```python
from build123d import *

# Parameters (mm, degrees)
SKETCH2_R           = 6.35
BOSS_EXTRUDE1_DEPTH = 19.05
SKETCH3_R           = 3.175
CUT_EXTRUDE1_DEPTH  = 20.05
SKETCH4_W           = 3.175
SKETCH4_H           = 0.79375
CHAMFER1_SIZE       = 0.396875
SKETCH5_W           = 3.020451336
SKETCH5_H           = 1.5875


with BuildPart() as part:
    # Sketch2 → Boss-Extrude1 (new body)
    with BuildSketch(Plane.XY):
        Circle(SKETCH2_R)
    extrude(amount=BOSS_EXTRUDE1_DEPTH)

    # Sketch3 → Cut-Extrude1 (cut, through all)
    with BuildSketch(Plane.XY.offset(19.05)):
        Circle(SKETCH3_R)
    extrude(amount=-CUT_EXTRUDE1_DEPTH, mode=Mode.SUBTRACT)

    # Sketch4 → Cut-Revolve1 (revolve, cut)
    with BuildSketch(Plane(origin=(0, 0, 0), x_dir=(1, 0, 0), z_dir=(0, 1, 0))):
        with Locations((6.329219641, -15.719425)):
            Rectangle(SKETCH4_W, SKETCH4_H)
        with Locations((6.329219641, -3.330575)):
            Rectangle(SKETCH4_W, SKETCH4_H)
    revolve(axis=Axis((0, 0, 19.05), (0, 0, -1)), mode=Mode.SUBTRACT)

    # Chamfer1
    chamfer1_edges = [part.edges().sort_by_distance(p)[0] for p in [
        (-6.35, 0, 0),
        (-6.35, 0, 19.05),
    ]]
    chamfer(chamfer1_edges, length=CHAMFER1_SIZE)

    # Sketch5 → Cut-Revolve2 (revolve, cut)
    with BuildSketch(Plane(origin=(0, 0, 0), x_dir=(1, 0, 0), z_dir=(0, 1, 0))):
        with Locations((6.35, -11.90625)):
            Rectangle(SKETCH5_W, SKETCH5_H)
        with Locations((6.35, -7.14375)):
            Rectangle(SKETCH5_W, SKETCH5_H)
    revolve(axis=Axis((0, 0, 19.05), (0, 0, -1)), mode=Mode.SUBTRACT)


solid = part.part
```
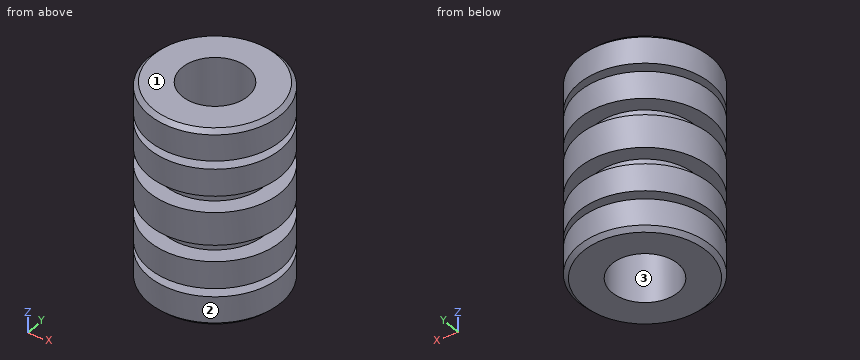
For this review, take the finished solid that the model builds, in its own axes (mm). Face numbers are marked on the shaded views. Round coordinates to 2 decimals unless told otherwise and drop trailing zeros. Write each loop counter-clockwise with the first axis right and the second up, starting at its lowest first coordinate (ties: lowest second). Pieces come first, ordered by that corner, then holes. Notation, with made-up numbers: (-15, 25.5) - (8, 25.5) arc R15 ccw to (8, 51.5) - close; hole circle Ø7 at (20, 41.5). An arc over 180 degrees is marked (long way). Answer as CSV lines item,"result". Start each with the question number.
(1) For pin 1 (3 mm diameter, centred on y = 2.5, z = 14, fed in from -X); pin 2 (1.5 mm diameter, centred on y = 4, z = 2.5, fed in from +X); pin 3 (1 mm diameter, centred on x = 5, z = 8.5, fed in from +Y), all flat-tipped, find the tip position at first contact; note any pin that passes through.
(2) Add section A-A, the plane z = 17.75. State the section outline as (x, y) points (3 decimals), plus the area to 3 significant figures.
(3) For line 1 (Z direction, x = 5.75, y = 1.5); line 2 (Y direction, x = 0, z = 15.25) (3 decimals); line 3 (Y direction, x = 0, z = 11.5) (3 decimals), list the stretches that pass through material, from the lowest coordinate up.
(4) Mouldability with a two-part tool opening along X and no side actions: class the marked faces 1, 2 and 3 as +X half, -X half, draft (parallel to the pull), parting line (faces both ways), or undercut.
(5) Add section B-B, the plane y = 5.25. State how many separate pieces and enclosed holes the cut face has, plus the area to 3 significant figures.
From the geometry:
1,pin 1,"stops at x = -6.27"
1,pin 2,"stops at x = 5.46"
1,pin 3,"stops at y = 4.48"
2,outline,"circle Ø12.7 at (0, 0); hole circle Ø6.35 at (0, 0)"
2,area,"95.0 mm²"
3,line 1,"z = 0 to 2.93, 3.73 to 6.35, 7.94 to 11.11, 12.7 to 15.32, 16.12 to 19.05"
3,line 2,"y = -6.35 to -3.175, 3.175 to 6.35"
3,line 3,"y = -4.84 to -3.175, 3.175 to 4.84"
4,face 1,"draft"
4,face 2,"parting line"
4,face 3,"undercut"
5,separate pieces,"5"
5,enclosed holes,"0"
5,area,"101 mm²"
